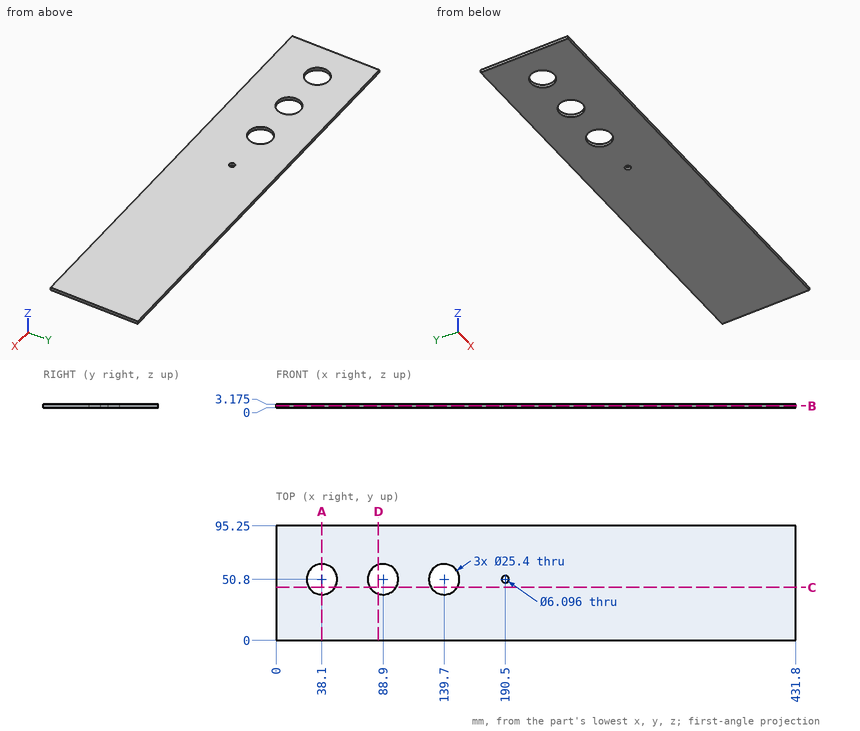
Drawing for the job (mm, zero at the part's lowest x, y, z). Round coordinates to 2 decimals unless told otherwise and drop trailing zeros. Write each loop counter-clockwise with the first axis right and the second up, starting at its lowest first coordinate (ties: lowest second). Pieces come first, ordered by that corner, then holes. Notation, with made-up numbers: M -6.5,54 L 25.5,54 A26 ccw 25.5,93 Z; hole C 48.25,17.5 d6. An arc over 180 degrees is marked long. Answer as a JSON object with one key per item and string values. Group by question number.
(1) Cut at B-B (z = 1.6). Give the cut face in (x, y).
(2) Drill centre lines: L1, parallel to Y at x = 88.9, z = 1.8; L2, parallel to Y at x = 190.5, z = 1.6; L3, parallel to X at y = 55, z = 0.8. Where is each one in solid material? Low to high.
(3) Cut at D-D (x = 85). Give the cut face in (y, z) (3 decimals), and give its area (3 significant figures).
(4) Cut at C-C (y = 44). Give the cut face in (x, z) (3 decimals), and give its area (3 significant figures).
(5) Cut at A-A (x = 38.1). Give the cut face in (y, z) (3 decimals).
Responses:
{
 "1": {"outline": "M 0,0 L 431.8,0 L 431.8,95.25 L 0,95.25 Z; hole C 38.1,50.8 d25.4; hole C 88.9,50.8 d25.4; hole C 139.7,50.8 d25.4; hole C 190.5,50.8 d6.1"},
 "2": {"L1": "y = 0 to 38.1, 63.5 to 95.25", "L2": "y = 0 to 47.75, 53.85 to 95.25", "L3": "x = 0 to 26.11, 50.09 to 76.91, 100.89 to 127.71, 151.69 to 431.8"},
 "3": {"outline": "M 0,0 L 38.714,0 L 38.714,3.175 L 0,3.175 Z; M 62.886,0 L 95.25,0 L 95.25,3.175 L 62.886,3.175 Z", "area": "226 mm2"},
 "4": {"outline": "M 0,0 L 27.374,0 L 27.374,3.175 L 0,3.175 Z; M 48.826,0 L 78.174,0 L 78.174,3.175 L 48.826,3.175 Z; M 99.626,0 L 128.974,0 L 128.974,3.175 L 99.626,3.175 Z; M 150.426,0 L 431.8,0 L 431.8,3.175 L 150.426,3.175 Z", "area": "1,170 mm2"},
 "5": {"outline": "M 0,0 L 38.1,0 L 38.1,3.175 L 0,3.175 Z; M 63.5,0 L 95.25,0 L 95.25,3.175 L 63.5,3.175 Z"}
}
